```python
from build123d import *

# Parameters (mm, degrees)
F0_R     = 11.1
F1_DEPTH = 7
F2_R     = 5
F3_R     = 5
F4_R     = 5


with BuildPart() as f1:
    # F0 (on Top) → F1 (new body)
    with BuildSketch(Plane.XY):
        with BuildLine():
            ThreePointArc((10.187081, 37.585558), (4.282363, 41.525705), (-2.589889, 43.304074))
            ThreePointArc((-2.589889, 43.304074), (-20.0319, 39.095625), (-32.678202, 26.367472))
            ThreePointArc((-32.678202, 26.367472), (-17.005905, 24.893365), (-3.464991, 16.866068))
            ThreePointArc((-3.464991, 16.866068), (-10.431292, 11.154526), (-18.783352, 7.779))
            ThreePointArc((-18.783352, 7.779), (-26.523062, 3.92607), (-32.973144, -1.831066))
            ThreePointArc((-32.973144, -1.831066), (-35.741861, -5.652046), (-37.643589, -9.970508))
            ThreePointArc((-37.643589, -9.970508), (-38.103497, -17.054217), (-36.207484, -23.894947))
            ThreePointArc((-36.207484, -23.894947), (-23.841854, -36.895947), (-6.4958, -41.483889))
            ThreePointArc((-6.4958, -41.483889), (-13.055333, -27.174228), (-12.873948, -11.433804))
            ThreePointArc((-12.873948, -11.433804), (-4.444456, -14.611027), (2.654864, -20.15636))
            ThreePointArc((2.654864, -20.15636), (9.861454, -24.932681), (18.072322, -27.640047))
            ThreePointArc((18.072322, -27.640047), (22.765746, -28.127337), (27.456508, -27.61505))
            ThreePointArc((27.456508, -27.61505), (33.821134, -24.471488), (38.797373, -19.409127))
            ThreePointArc((38.797373, -19.409127), (43.873754, -2.199678), (39.174002, 15.116417))
            ThreePointArc((39.174002, 15.116417), (30.061239, 2.280864), (16.338939, -5.432264))
            ThreePointArc((16.338939, -5.432264), (14.875749, 3.456501), (16.128488, 12.37736))
            ThreePointArc((16.128488, 12.37736), (16.661608, 21.00661), (14.900822, 29.471114))
            ThreePointArc((14.900822, 29.471114), (12.976115, 33.779383), (10.187081, 37.585558))
        make_face()
        with Locations((-25.980762, -15)):
            Circle(F0_R, mode=Mode.SUBTRACT)
        Circle(F0_R, mode=Mode.SUBTRACT)
        with Locations((25.980762, -15)):
            Circle(F0_R, mode=Mode.SUBTRACT)
        with Locations((0, 30)):
            Circle(F0_R, mode=Mode.SUBTRACT)
    extrude(amount=F1_DEPTH)

    # F2
    f2_edges = [f1.edges().sort_by_distance(p)[0] for p in [
        (16.338939, -5.432264, 3.5),
    ]]
    fillet(f2_edges, radius=F2_R)

    # F3
    f3_edges = [f1.edges().sort_by_distance(p)[0] for p in [
        (-3.464991, 16.866068, 3.5),
    ]]
    fillet(f3_edges, radius=F3_R)

    # F4
    f4_edges = [f1.edges().sort_by_distance(p)[0] for p in [
        (-12.873948, -11.433804, 3.5),
    ]]
    fillet(f4_edges, radius=F4_R)


solid = f1.part
```
Input: part model. Units: mm. Frame: model coordinates. A direction names the side the tool comes from. Give positions to 0.01 mm unless a question says otherwise; leave off trailing zeros. Loops run counter-clockwise (first coordinate to the right, second up) from the corner with the lowest first, then second, coordinate; pieces in that order, holes last. Notation, with made-up numbers: M 23.25,26.5 L 78.25,26.5 A19 ccw 78.25,37.5 Z; hole C -1,62 d11. An arc over 180 degrees is marked long. Answer as CSV lines item,"result". Start each with the question number.
1. Section A-A on x = 33. Return loops of the section in (y, z).
2. Section C-C on x = 0. Return loops of the section in (y, z), plus the area to 3 significant figures.
3. Pull-direction query (Y, two-part tool) for faces 4 (the face through (4.373, 41.485, 3.451)), 5 (the face through (5.97, 9.36, 3.45)), 6 (the face through (-24.06, -36.766, 3.451)); classes: released by +Y, released by -Y, zero draft, split by the parting line, or undercut.
4. Pin query (flat end, axial travel): P1, Ø3, axis at x = -25, z = 5.5, coming from the +Y side; P2, Ø1, axis at y = -2, z = 6, coming from the -X side. Return the tip coordinate at first contact, or that it passes through.
5. Line query: L1, parallel to Y at x = 0, z = 2; L2, parallel to X at y = -7.5, z = 1; L3, parallel to X at y = 1, z = 2.5. Output: solid intervals per line, ascending.
6. Section B-B on y = 5. Return loops of the section in (x, z), plus the area to 3 significant figures.
7. Section D-D on z = 1. State how many separate pieces and enclosed holes the cut face has, plus the area to 3 significant figures.
8. Reachability of faces 1 (the face through (-12.204, -30.428, 3.451)), 2 (the face through (10, -25, 3)), 3 (the face through (32.45, 4.64, 3.45)) from +Z, -Z, +X, -X, +Y, -Y: full face, straight path, thin tool, end or side. Return the list, or none.
Computed values:
1,outline,"M -25.04,0 L -23.6,0 L -23.6,7 L -25.04,7 Z; M -6.4,0 L 5.25,0 L 5.25,7 L -6.4,7 Z"
2,outline,"M -17.67,0 L -11.1,0 L -11.1,7 L -17.67,7 Z; M 11.1,0 L 18.9,0 L 18.9,7 L 11.1,7 Z; M 41.1,0 L 42.92,0 L 42.92,7 L 41.1,7 Z"
2,area,"113 mm²"
3,face 4,"released by +Y"
3,face 5,"undercut"
3,face 6,"released by -Y"
4,P1,"stops at y = 36.85"
4,P2,"stops at x = -33.55"
5,L1,"y = -17.67 to -11.1, 11.1 to 18.9, 41.1 to 42.92"
5,L2,"x = -36.69 to -34.16, -17.8 to -8.18, 8.18 to 17.8, 34.16 to 43.39"
5,L3,"x = -30.23 to -11.05, 11.05 to 15.01, 28.56 to 43.75"
6,outline,"M -24.83,0 L -9.91,0 L -9.91,7 L -24.83,7 Z; M 9.91,0 L 14.9,0 L 14.9,7 L 9.91,7 Z; M 32.78,0 L 43.16,0 L 43.16,7 L 32.78,7 Z"
6,area,"212 mm²"
7,separate pieces,"1"
7,enclosed holes,"4"
7,area,"2,040 mm²"
8,face 1,"+Z, -Z"
8,face 2,"+Z, -Z, -Y"
8,face 3,"+Z, -Z, +Y"
